```python
from build123d import *

# Parameters (mm, degrees)
SKETCH1_R           = 6
BOSS_EXTRUDE1_DEPTH = 2
SKETCH2_R           = 2
BOSS_EXTRUDE2_DEPTH = 35
FILLET1_R           = 2
CUT_EXTRUDE1_START  = -5
SKETCH4_R           = 2
CUT_EXTRUDE1_DEPTH  = 5


with BuildPart() as part:
    # Sketch1 → Boss-Extrude1 (new body)
    with BuildSketch(Plane.XY):
        Circle(SKETCH1_R)
    extrude(amount=BOSS_EXTRUDE1_DEPTH)

    # Sketch2 → Boss-Extrude2 (add)
    with BuildSketch(Plane.XY.offset(2)):
        Circle(SKETCH2_R)
    extrude(amount=BOSS_EXTRUDE2_DEPTH)

    # Fillet1
    fillet1_edges = [part.edges().sort_by_distance(p)[0] for p in [
        (-2, 0, 2),
    ]]
    fillet(fillet1_edges, radius=FILLET1_R)

    # Sketch4 → Cut-Extrude1 (cut)
    with BuildSketch(Plane.XY.offset(37).offset(CUT_EXTRUDE1_START)):
        Circle(SKETCH4_R)
    extrude(amount=CUT_EXTRUDE1_DEPTH, mode=Mode.SUBTRACT)


solid = part.part
```
Source: CAD feature listing. Evaluate the final solid. Frame: model axes, mm. A direction names the side the tool comes from. Round coordinates to 2 decimals unless told otherwise and drop trailing zeros. Loops run counter-clockwise (first coordinate to the right, second up) from the corner with the lowest first, then second, coordinate; pieces in that order, holes last. Notation, with made-up numbers: M 30,-2.5 L 81,-2.5 A14 ccw 81,16.5 Z; hole C 4.25,43 d5. An arc over 180 degrees is marked long. Use a Markdown table: item, result. Add a question column.
1. Set-up query: faces 1 (the flat face through (-1.42, -3.92, 2)), 2 (the flat face through (0, 0, 0)). Return all of +Z, -Z, +X, -X, +Y, -Y with unobstructed straight access to the full face (end or side cutting, diameter ignored); none if empty.
2. Cut plane C-C, the plane z = 22. Output: boundary loops of the cut face in (x, y).
3. Ray query, line 1 along Z through (x, y) = (-1.25, -4.5); line 2 along Y through (x, z) = (-1, 3); line 3 along Z through (x, y) = (-2.5, 0). Return the intervals inside material, ascending. Write a range as [from, to].
4. Cut plane A-A, the plane y = 0. Output: boundary loops of the cut face in (x, z), and give its area (3 significant figures).
5. Contact query for flat-ended pins moving along their axis: pin 1 (5 mm diameter, centred on x = -1, z = 17.5, fed in from +Y); pin 2 (4 mm diameter, centred on x = 2.5, z = 19, fed in from +Y); pin 3 (4 mm diameter, centred on x = -1, z = 25.5, fed in from -Y). Output: stop coordinate, or through.
Solution:
| question | item | result |
|---|---|---|
| 1 | face 1 | +Z |
| 1 | face 2 | -Z, +X, -X, +Y, -Y |
| 2 | outline | C 0,0 d4 |
| 3 | line 1 | z = [0, 2] |
| 3 | line 2 | y = [-2.04, 2.04] |
| 3 | line 3 | z = [0, 2.68] |
| 4 | outline | M -6,0 L 6,0 L 6,2 L 4,2 A2 cw 2,4 L 2,32 L -2,32 L -2,4 A2 cw -4,2 L -6,2 Z |
| 4 | area | 146 mm2 |
| 5 | pin 1 | stops at y = 2 |
| 5 | pin 2 | stops at y = 1.94 |
| 5 | pin 3 | stops at y = -2 |
